```python
from build123d import *

# Parameters (mm, degrees)
SKETCH1_W           = 34
SKETCH1_H           = 54
SKETCH1_W_2         = 10
SKETCH1_H_2         = 3
SKETCH1_W_3         = 1
SKETCH1_H_3         = 7
SKETCH1_H_4         = 20
BOSS_EXTRUDE1_DEPTH = 3


with BuildPart() as part:
    # Sketch1 → Boss-Extrude1 (new body)
    with BuildSketch(Plane(origin=(0, 0, 0), x_dir=(1, 0, 0), z_dir=(0, 1, 0))):
        with Locations((18, 30)):
            Rectangle(SKETCH1_W, SKETCH1_H)
        with Locations((10, 1.5)):
            Rectangle(SKETCH1_W_2, SKETCH1_H_2)
        with Locations((26, 1.5)):
            Rectangle(SKETCH1_W_2, SKETCH1_H_2)
        with Locations((35.5, 6.5)):
            Rectangle(SKETCH1_W_3, SKETCH1_H_3)
        with Locations((35.5, 30)):
            Rectangle(SKETCH1_W_3, SKETCH1_H_4)
        with Locations((35.5, 53.5)):
            Rectangle(SKETCH1_W_3, SKETCH1_H_3)
        with Locations((26, 58.5)):
            Rectangle(SKETCH1_W_2, SKETCH1_H_2)
        with Locations((10, 58.5)):
            Rectangle(SKETCH1_W_2, SKETCH1_H_2)
        with Locations((0.5, 53.5)):
            Rectangle(SKETCH1_W_3, SKETCH1_H_3)
        with Locations((0.5, 30)):
            Rectangle(SKETCH1_W_3, SKETCH1_H_4)
        with Locations((0.5, 6.5)):
            Rectangle(SKETCH1_W_3, SKETCH1_H_3)
    extrude(amount=BOSS_EXTRUDE1_DEPTH)


solid = part.part
```
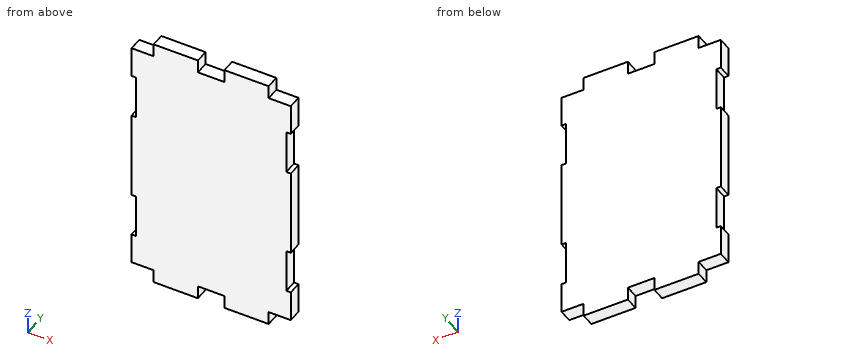
CAD build for the part. Positions are in the model's coordinates, mm. Give positions to 0.01 mm unless a question says otherwise; leave off trailing zeros. Write each loop counter-clockwise with the first axis right and the second up, starting at its lowest first coordinate (ties: lowest second). Pieces come first, ordered by that corner, then holes. Notation, with made-up numbers: M -4,85 L 38,85 A20 ccw 38,93 Z; hole C 64,28 d1. An arc over 180 degrees is marked long. Return JSON: item names as keys, results as strings. Group by question number.
(1) Band-saw the part on B-B (z = -48.5). Give the cut face in (x, y), and give its area (3 significant figures).
(2) Drill centre lines: L1, parallel to X at y = 1.7, z = -2.5; L2, parallel to Z at x = 2.5, y = 1.8; L3, parallel to X at y = 0.95, z = -46. Where is each one in solid material? Low to high. Write a range as [from, to].
(3) Band-saw the part on A-A (x = 4). Give the cut face in (y, z).
(4) Flat gauge pins, fed straight in: pin 1 Ø1.5 at (y, z) = (1, -1) entering from -X; pin 2 Ø0.9 at (y, z) = (1.5, -15) entering from +X; pin 3 Ø0.5 at (x, y) = (35.5, 1.5) entering from -Z. Where does each tip first touch, or does it go through?
Entries:
{
 "1": {"outline": "M 1,0 L 35,0 L 35,3 L 1,3 Z", "area": "102 mm^2"},
 "2": {"L1": "x = [5, 15], [21, 31]", "L2": "z = [-57, -3]", "L3": "x = [1, 35]"},
 "3": {"outline": "M 0,-57 L 3,-57 L 3,-3 L 0,-3 Z"},
 "4": {"pin 1": "stops at x = 5", "pin 2": "stops at x = 35", "pin 3": "stops at z = -57"}
}
